```python
from build123d import *

# Parameters (mm, degrees)
F0_W     = 101.6
F0_H     = 101.6
F1_DEPTH = 50.8
F2_R     = 25.4
F3_DEPTH = 101.601
F4_R     = 25.4
F5_DEPTH = 101.601
F6_R     = 25.4
F7_DEPTH = 101.601


with BuildPart() as f1:
    # F0 (on Front) → F1 (new body, symmetric)
    with BuildSketch(Plane.XZ):
        Rectangle(F0_W, F0_H)
    extrude(amount=F1_DEPTH, both=True)

    # F2 (on face) → F3 (cut, through all)
    with BuildSketch(Plane.XY.offset(50.8)):
        Circle(F2_R)
    extrude(amount=-F3_DEPTH, mode=Mode.SUBTRACT)

    # F4 (on face) → F5 (cut, through all)
    with BuildSketch(Plane.XZ.offset(50.8)):
        Circle(F4_R)
    extrude(amount=-F5_DEPTH, mode=Mode.SUBTRACT)

    # F6 (on face) → F7 (cut, through all)
    with BuildSketch(Plane.YZ.offset(50.8)):
        Circle(F6_R)
    extrude(amount=-F7_DEPTH, mode=Mode.SUBTRACT)


solid = f1.part
```
For this review, take the finished solid that the model builds, in its own axes (mm). Give positions to 0.01 mm unless a question says otherwise; leave off trailing zeros. Write each loop counter-clockwise with the first axis right and the second up, starting at its lowest first coordinate (ties: lowest second). Pieces come first, ordered by that corner, then holes.
Item 1: Take a section at B-B (x = -20). Give the boundary of the cut face in (y, z), and give its area (3 significant figures).
Item 2: Insertion check: P1, Ø12, axis at x = 0.5, y = 22.5, coming from the +Z side. The pin has a flat end and moves straight along its axis. Give the tip position at first contact, or say it passes through.
Item 3: Take a section at A-A (y = 0). Give the boundary of the cut face in (x, z), and give its area (3 significant figures).
Item 4: The part is to be moulded in two halves that separate along Z. For faces 1 (the face through (-12, -23, -50.8)), 2 (the face through (-18.72, 37.8, 17.17)), 3 (the face through (-18.72, -38.26, 17.17)), 4 (the face through (50.8, -23, -12)), say which applies: +Z half, -Z half, draft (parallel to the pull), parting line (faces both ways), or undercut.
Item 5: Wall thickness on probe 1 along Z at (x, y) = (0, 35); probe 2 along Z at (x, y) = (43.5, 12); probe 3 along X at (y, z) = (3, 26): over which ranges is each line inside the solid? List them lowest first.
Item 6: Take a section at D-D (z = 44.5). Give the boundary of the cut face in (x, y), and give its area (3 significant figures).
Established:
1. outline: (-50.8, -50.8) - (-15.66, -50.8) - (-15.66, -20) arc R25.4 cw to (-20, -15.66) - (-50.8, -15.66) - close; (-50.8, 15.66) - (-20, 15.66) arc R25.4 cw to (-15.66, 20) - (-15.66, 50.8) - (-50.8, 50.8) - close; (15.66, -50.8) - (50.8, -50.8) - (50.8, -15.66) - (20, -15.66) arc R25.4 cw to (15.66, -20) - close; (15.66, 20) arc R25.4 cw to (20, 15.66) - (50.8, 15.66) - (50.8, 50.8) - (15.66, 50.8) - close
1. area: 4,900 mm2
2. P1: stops at z = 50.8
3. outline: (-50.8, -50.8) - (-25.4, -50.8) - (-25.4, -25.4) - (-50.8, -25.4) - close; (-50.8, 25.4) - (-25.4, 25.4) - (-25.4, 50.8) - (-50.8, 50.8) - close; (25.4, -50.8) - (50.8, -50.8) - (50.8, -25.4) - (25.4, -25.4) - close; (25.4, 25.4) - (50.8, 25.4) - (50.8, 50.8) - (25.4, 50.8) - close
3. area: 2,580 mm2
4. face 1: -Z half
4. face 2: undercut
4. face 3: undercut
4. face 4: draft
5. probe 1: z = -50.8 to -25.4, 25.4 to 50.8
5. probe 2: z = -50.8 to -22.39, 22.39 to 50.8
5. probe 3: x = -50.8 to -25.22, 25.22 to 50.8
6. outline: (-50.8, -50.8) - (50.8, -50.8) - (50.8, 50.8) - (-50.8, 50.8) - close; hole circle Ø50.8 at (0, 0)
6. area: 8,300 mm2
